Autodesk Inventor part; units mm, degrees
ref_plane "YZ Plane" through (0, 0, 0) normal (1, 0, 0) x (0, 1, 0)
ref_plane "XZ Plane" through (0, 0, 0) normal (0, 1, 0) x (-1, 0, 0)
ref_plane "XY Plane" through (0, 0, 0) normal (0, 0, 1) x (1, 0, 0)
sketch "Sketch1" plane through (0, 0, 0) normal (0, 0, 1) x (1, 0, 0)
  line L0 (-100, 100) -> (100, 100)
  line L1 (100, 100) -> (100, 0)
  line L2 (100, 0) -> (-100, 0)
  line L3 (-100, 0) -> (-100, 100)
  arc A0 (77.5, 0) -> (2.5, 0) centre (40, 11.6402) ccw
  point P0 (0, 0)
  point P1 (0, 100)
  point P2 (0, 0)
  dimension "d0" = 200
  dimension "d1" = 100
  dimension "d22" = 75
  dimension "d23" = 102.5
extrude "Extrusion1" add sketch "Sketch1" along normal blind 4 contours L0 L1 L2 A0 L3
sketch "Sketch2" plane through (0, 0, 4) normal (0, 0, 1) x (1, 0, 0)
  line L0 (-100, 100) -> (-100, 0)
  line L1 (-100, 0) -> (-96, 0)
  line L2 (-96, 0) -> (-96, 35)
  line L3 (-96, 35) -> (-100, 35)
  line L4 (-100, 35) -> (-100, 0)
  line L5 (-100, 100) -> (-96, 100)
  line L6 (-96, 100) -> (-96, 65)
  line L7 (-96, 65) -> (-100, 65)
  line L8 (-100, 65) -> (-100, 100)
  point P0 (0, 0)
  dimension "d9" = 4
  dimension "d10" = 35
  dimension "d11" = 4
  dimension "d12" = 35
extrude "Extrusion2" cut sketch "Sketch2" against normal through all
sketch "Sketch3" plane through (-24.1746, 0, 0) normal (0, -1, 0) x (1, 0, 0)
  line L0 (-71.8254, 4) -> (124.1746, 4)
  line L1 (-55.8254, 4) -> (-5.8254, 4)
  line L2 (-5.8254, 4) -> (-5.8254, 0)
  line L3 (-5.8254, 0) -> (-55.8254, 0)
  line L4 (-55.8254, 0) -> (-55.8254, 4)
  line L5 (-75.8254, 0) -> (-75.8254, 4)
  line L6 (124.1746, 0) -> (-71.8254, 0)
  line L7 (124.1746, 4) -> (-71.8254, 4)
  line L8 (124.1746, 0) -> (124.1746, 4)
  point P0 (24.1746, 0)
  point P1 (0, 4)
  point P2 (117.1746, 0)
  point P3 (105.1746, 4)
  point P4 (-5.8254, 4)
  dimension "d15" = 4
  dimension "d16" = 20
  dimension "d17" = 50
extrude "Extrusion3" add sketch "Sketch3" along normal blind 4 contours L0 L2 L3 L4
sketch "Sketch5" plane through (100, 0, 0) normal (1, 0, 0) x (0, 0, -1)
  line L0 (-4, 100) -> (-4, 65)
  line L1 (-4, 100) -> (0, 100)
  line L2 (0, 100) -> (0, 0)
  line L3 (0, 0) -> (-4, 0)
  line L4 (-4, 0) -> (-4, 100)
extrude "Extrusion5" add sketch "Sketch5" along normal blind 80
sketch "Sketch6" plane through (0, 0, 4) normal (0, 0, 1) x (1, 0, 0)
  line L0 (-96, 100) -> (180, 100)
  line L1 (180, 100) -> (19, 100)
  line L2 (180, 100) -> (180, 0)
  line L3 (180, 100) -> (180, -12.7334)
  line L4 (180, -12.7334) -> (19, 100)
  point P0 (0, 0)
  dimension "d30" = 35
  dimension "d33" = 115
extrude "Extrusion6" cut sketch "Sketch6" against normal blind 80
sketch "Sketch7" plane through (161.8148, 0, 4) normal (0.5735764, 0.819152, 0) x (0.819152, -0.5735764, 0)
  line L0 (0, 0) -> (-174.3447, 0)
  line L1 (-69.0666, 4) -> (-145.7265, 4)
  line L2 (-63, 0) -> (-113, 0)
  line L3 (-113, 0) -> (-113, 4)
  line L4 (-113, 4) -> (-63, 4)
  line L5 (-63, 4) -> (-63, 0)
  line L6 (0, 4) -> (0, 0)
  line L7 (-113, 0) -> (-151, 0)
  line L8 (-151, 0) -> (-151, 4)
  line L9 (-151, 4) -> (-113, 4)
  line L10 (-113, 4) -> (-113, 0)
  point P0 (-132.5509, 4)
  point P1 (-130.503, 4)
  point P2 (0, 2)
  point P3 (-63, 2)
  point P4 (-113, 0)
  point P5 (-151, 0)
  dimension "d34" = 50
  dimension "d35" = 63
  dimension "d56" = 38
extrude "Extrusion7" cut sketch "Sketch7" against normal blind 4
sketch "Sketch8" plane through (-96, 100, 4) normal (0, 1, 0) x (1, 0, 0)
  line L0 (112, 4) -> (0, 4)
  line L1 (63, 0) -> (80.5, 0)
  line L2 (30.5, 4) -> (80.5, 4)
  line L3 (80.5, 4) -> (80.5, 0)
  line L4 (80.5, 0) -> (30.5, 0)
  line L5 (30.5, 0) -> (30.5, 4)
  line L6 (0, 4) -> (0, 0)
  line L7 (0, 4) -> (0, 0)
  point P0 (96, 4)
  point P1 (80.5, 2)
  point P2 (30.5, 2)
  point P3 (80.5, 4)
  point P4 (0, 2)
  point P5 (0, 2)
  dimension "d38" = 50
  dimension "d42" = 30.5
extrude "Extrusion8" cut sketch "Sketch8" against normal blind 4
sketch "Sketch9" plane through (161.8148, 0, 4) normal (0.5735764, 0.819152, 0) x (0.819152, -0.5735764, 0)
  line L0 (-63, 4) -> (0, 4)
  line L1 (0, 0) -> (-63, 0)
  line L2 (0, 4) -> (-7.082, 4)
  line L3 (-7.082, 4) -> (-7.082, 0)
  line L4 (-7.082, 0) -> (0, 0)
  line L5 (0, 0) -> (0, 4)
  point P0 (-132.5509, 4)
  point P1 (-7.082, 4)
  dimension "d43" = 7.082
extrude "Extrusion9" cut sketch "Sketch9" against normal through all
sketch "Sketch10" plane through (77.5, 0, 0) normal (0, -1, 0) x (1, 0, 0)
  line L0 (30.4139, 4) -> (-41.6715, 4)
  line L1 (32.7082, 0) -> (78.5136, 0)
  line L2 (25, 4) -> (55, 4)
  line L3 (55, 4) -> (55, 0)
  line L4 (55, 0) -> (25, 0)
  line L5 (25, 0) -> (25, 4)
  line L6 (0, 0) -> (0, 4)
  point P0 (-77.5, 0)
  point P1 (-10.5437, 4)
  point P2 (25, 2)
  point P3 (0, 2)
  dimension "d46" = 30
  dimension "d47" = 25
extrude "Extrusion10" add sketch "Sketch10" along normal blind 4
sketch "Sketch11" plane through (0, 0, 0) normal (0, 0, -1) x (-1, 0, 0)
  line L0 (16, 54) -> (66, 54)
  line L1 (66, 54) -> (66, 50)
  line L2 (66, 50) -> (16, 50)
  line L3 (16, 50) -> (16, 54)
  line L4 (96, 0) -> (96, 35)
  point P0 (0, 0)
  point P1 (41, 50)
  dimension "d50" = 50
  dimension "d51" = 4
  dimension "d52" = 55
  dimension "d53" = 50
extrude "Extrusion11" cut sketch "Sketch11" against normal blind 4
sketch "Sketch15" plane through (0, 0, 4) normal (0, 0, 1) x (1, 0, 0)
  line L0 (107.9139, 32.8587) -> (35.8285, 83.3334)
  line L1 (107.9139, 32.8587) -> (100.9511, 37.7341)
  line L2 (110.2082, 36.1353) -> (107.9139, 32.8587)
  line L3 (107.9139, 32.8587) -> (112.6172, 39.5758)
  line L4 (110.2082, 36.1353) -> (113.4848, 33.841)
  line L5 (156.0136, 4.0621) -> (110.2082, 36.1353)
  line L6 (112.6172, 39.5758) -> (115.8939, 37.2814)
  line L7 (115.8939, 37.2814) -> (113.4848, 33.841)
  line L8 (112.6172, 39.5758) -> (83.9469, 59.6509)
  line L9 (83.9469, 59.6509) -> (81.6526, 56.3743)
  line L10 (81.6526, 56.3743) -> (110.3229, 36.2991)
  line L11 (115.8939, 37.2814) -> (156.0136, 4.0621)
  point P0 (0, 0)
  point P1 (120.2672, 29.092)
  dimension "d61" = 8.2
  dimension "d62" = 4
  dimension "d63" = 35
  dimension "d64" = 4
extrude "Extrusion12" add sketch "Sketch15" against normal blind 4
sketch "Sketch16" plane through (77.5, -4, 0) normal (0, -1, 0) x (1, 0, 0)
  line L0 (55, 0) -> (55, 4)
  line L1 (25, 0) -> (55, 0)
  line L2 (55, 4) -> (25, 4)
  line L3 (25, 4) -> (25, 0)
  line L4 (25, 0) -> (55, 0)
  line L5 (55, 0) -> (55, 4)
  point P0 (-77.5, 0)
extrude "Extrusion13" add sketch "Sketch16" along normal blind 8.3
sketch "Sketch17" plane through (0, 0, 4) normal (0, 0, 1) x (1, 0, 0)
  line L0 (77.5, 0) -> (102.5, 0)
  line L1 (102.5, 0) -> (102.5, -12.3)
  line L2 (102.5, -4) -> (112.5, -4)
  line L3 (112.5, -4) -> (112.5, -8.1)
  line L4 (112.5, -8.1) -> (102.5, -8.1)
  line L5 (102.5, -8.1) -> (102.5, -4)
  line L6 (132.5, -12.3) -> (102.5, -12.3)
  line L7 (117.5, -12.3) -> (132.5, -12.3)
  line L8 (132.5, -12.3) -> (132.5, 0)
  line L9 (132.5, -4) -> (116.0511, -12.3)
  point P0 (0, 0)
  dimension "d71" = 4
  dimension "d72" = 4.1
  dimension "d73" = 4.2
  dimension "d74" = 10
  dimension "d77" = 4
extrude "Extrusion14" cut sketch "Sketch17" against normal blind 8.3
sketch "Sketch21" plane through (0, 0, 4) normal (0, 0, 1) x (1, 0, 0)
  line L0 (-80, -4) -> (-100, -4)
  line L1 (-100, -4) -> (-100, -8)
  line L2 (-100, -8) -> (-80, -8)
  line L3 (-80, -8) -> (-80, -4)
  line L4 (-80, -4) -> (-30, -4)
  line L5 (-30, -4) -> (-30, -8)
  line L6 (-30, -8) -> (-80, -8)
  line L7 (-80, -8) -> (-80, -4)
  line L8 (-30, -4) -> (-30, -4)
  line L9 (-30, -8) -> (-14, -8)
  line L10 (-30, -4) -> (-14, -4)
  line L11 (-14, -4) -> (-14, -8)
  line L12 (-14, -8) -> (-30, -8)
  line L13 (-30, -8) -> (-30, -4)
  point P0 (0, 0)
  dimension "d80" = 20
  dimension "d81" = 4
  dimension "d82" = 50
  dimension "d85" = 16
extrude "Extrusion15" add sketch "Sketch21" against normal blind 4
properties part number "Tapa lateral 1"
Geometry check sheet. Reference: the model listing, model coordinates, mm. A direction names the side the tool comes from. Coordinates: 2 decimals unless noted, no trailing zeros. Write each loop counter-clockwise with the first axis right and the second up, starting at its lowest first coordinate (ties: lowest second). Pieces come first, ordered by that corner, then holes. Notation, with made-up numbers: (-4, 0) -> (27, 0) arc R27 ccw to (27, 21) -> close; hole circle Ø10 at (68.25, 36). An arc over 180 degrees is marked (long way). Use CSV: the item, a comma, the result in double quotes. Start each with the question number.
Item 1: Mould release check, pull along Y, two halves, no side actions. Record for faces 3 (the flat face through (-2, 45, 4)), 4 (the flat face through (124.391, -8.092, 2.028)), 5 (the flat face through (95.787, 46.477, 2.028)): released by +Y, released by -Y, zero draft, split by the parting line, or undercut.
Item 2: Cross-section at A-A, the plane x = -60. Record the cut outline in (y, z).
Item 3: Set-up check for faces 1 (the flat face through (135.673, 20.904, 2.028)), 2 (the flat face through (71.365, 58.448, 1.972)): record each of +Z, -Z, +X, -X, +Y, -Y from which the full face is reachable in a straight line by a thin tool's end or side.
Item 4: Depth check by flat-ended pin: pin 1 Ø10 at (x, y) = (-53, 73) entering from -Z; pin 2 Ø1.2 at (y, z) = (-6.5, 2.5) entering from +X; pin 3 Ø1.2 at (x, z) = (-31, 1) entering from -Y; pin 4 Ø2 at (x, z) = (-98.5, 2) entering from +Y. Enter the tip coordinate at first touch or a pass-through.
Item 5: Cross-section at B-B, the plane y = 28. Record the cut outline in (x, z).
Item 6: Cross-section at C-C, the plane x = 45.5. Record the cut outline in (y, z), plus the area to 3 significant figures.
Item 7: Thickness scan on line 1 (X direction, y = 53, z = 0.85); line 2 (Y direction, x = -80.5, z = 2.15); line 3 (X direction, y = 33, z = 2.5). Record the ranges inside material, lowest first.
Answers:
1,face 3,"zero draft"
1,face 4,"released by -Y"
1,face 5,"undercut"
2,outline,"(-8, 0) -> (50, 0) -> (50, 4) -> (-8, 4) -> close; (54, 0) -> (96, 0) -> (96, 4) -> (54, 4) -> close"
3,face 1,"+Z, -Z, +X, +Y"
3,face 2,"+Z, -Z"
4,pin 1,"z = 0"
4,pin 2,"x = 128.73"
4,pin 3,"y = -8"
4,pin 4,"y = 65"
5,outline,"(-96, 0) -> (4.31, 0) -> (4.31, 4) -> (-96, 4) -> close; (75.69, 0) -> (127.1, 0) -> (127.1, 4) -> (75.69, 4) -> close"
6,outline,"(50.52, 0) -> (76.56, 0) -> (76.56, 4) -> (50.52, 4) -> close"
6,area,"104 mm^2"
7,line 1,"-100 to -66, -16 to 79.15, 86.47 to 93.45"
7,line 2,"-8 to -4, 0 to 100"
7,line 3,"-96 to 7.05, 72.95 to 107.71, 108.01 to 121.06"
